Read the model definition and answer for the solid it produces. Units are mm, in the model's axes. Face numbers are marked on the shaded views. A direction names the side the tool comes from. Give positions to 0.01 mm unless a question says otherwise; leave off trailing zeros. Order: outer loops, then holes, each group sorted by start corner. A loop starts at its lowest first (then second) coordinate and runs counter-clockwise, first axis right, second up.
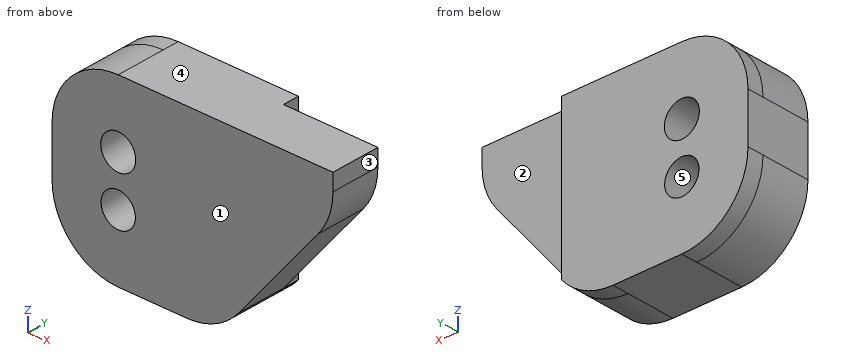
```python
from build123d import *

# Parameters (mm, degrees)
BOSS_EXTRUDE1_DEPTH = 19.05
FILLET1_R           = 25.4
BOSS_EXTRUDE2_DEPTH = 6.35
SKETCH4_R           = 6.721788933
SKETCH4_R_2         = 6.590945077
CUT_EXTRUDE3_DEPTH  = 26.4


with BuildPart() as part:
    # Sketch1 → Boss-Extrude1 (new body)
    with BuildSketch(Plane(origin=(0, 0, 0), x_dir=(1, 0, 0), z_dir=(0, 1, 0))):
        Polygon((10.04026689, 34.907603773), (53.917892581, -19.499033471), (53.917892581, -34.907603773), (-53.917892581, -34.907603773), (-53.917892581, 34.907603773), align=None)
    extrude(amount=BOSS_EXTRUDE1_DEPTH)

    # Fillet1
    fillet1_edges = [part.edges().sort_by_distance(p)[0] for p in [
        (-53.917892581, 9.525, -34.907603773),
        (10.04026689, 9.525, -34.907603773),
        (53.917892581, 9.525, 19.499033471),
        (-53.917892581, 9.525, 34.907603773),
    ]]
    fillet(fillet1_edges, radius=FILLET1_R)

    # Sketch3 → Boss-Extrude2 (add)
    with BuildSketch(Plane(origin=(0, 19.05, 0), x_dir=(1, 0, 0), z_dir=(0, 1, 0))):
        with BuildLine():
            Line((17.665332694, 25.452803459), (17.665332694, -34.907603773))
            Line((17.665332694, -34.907603773), (-28.517892581, -34.907603773))
            ThreePointArc((-28.517892581, -34.907603773), (-46.478404823, -27.468116015), (-53.917892581, -9.507603773))
            Line((-53.917892581, -9.507603773), (-53.917892581, 9.507603773))
            ThreePointArc((-53.917892581, 9.507603773), (-46.478404823, 27.468116015), (-28.517892581, 34.907603773))
            Line((-28.517892581, 34.907603773), (-2.106126711, 34.907603773))
            ThreePointArc((-2.106126711, 34.907603773), (8.851791157, 32.422315991), (17.665332694, 25.452803459))
        make_face()
    extrude(amount=BOSS_EXTRUDE2_DEPTH)

    # Sketch4 → Cut-Extrude3 (cut, through all)
    with BuildSketch(Plane(origin=(0, 25.4, 0), x_dir=(1, 0, 0), z_dir=(0, 1, 0))):
        with Locations(Location((-28.517892581, -9.507603773, 0), (0, 0, 270))):  # turned: the seam where the file's is
            Circle(SKETCH4_R)
        with Locations(Location((-28.517892581, 9.507603773, 0), (0, 0, 270))):  # turned: the seam where the file's is
            Circle(SKETCH4_R_2)
    extrude(amount=-CUT_EXTRUDE3_DEPTH, mode=Mode.SUBTRACT)


solid = part.part
```
1) The part is cut by section B-B on z = 19.5. Determine the outline of the cut face in (x, y), and give its area (3 significant figures).
Final values:
outline: (-51.87, 0) - (52.28, 0) - (52.28, 19.05) - (17.67, 19.05) - (17.67, 25.4) - (-51.87, 25.4) - close
area: 2,430 mm2
2) Given pin 1 (11 mm diameter, centred on x = 39.5, z = 5.5, fed in from +Y); pin 2 (1.9 mm diameter, centred on y = 21.5, z = 8, fed in from +X); pin 3 (12 mm diameter, centred on x = -28.52, z = 9.51, fed in from +Y); pin 4 (2 mm diameter, centred on y = 7, z = 22, fed in from +X), each flat-ended and moving along its own axis, determine where each tip first touches the part or whether it passes through.
Final values:
pin 1: stops at y = 19.05
pin 2: stops at x = 17.67
pin 3: passes through
pin 4: stops at x = 53.32
3) The part is cut by section C-C on x = 13. Determine the outline of the cut face in (y, z), and give its area (3 significant figures).
Final values:
outline: (0, -29.93) - (25.4, -29.93) - (25.4, 34.91) - (0, 34.91) - close
area: 1,650 mm2
4) The part is cut by section A-A on y = 2. Determine the outline of the cut face in (x, z), and give its area (3 significant figures).
Final values:
outline: (-53.92, -9.51) arc R25.4 ccw to (-28.52, -34.91) - (-2.11, -34.91) arc R25.4 ccw to (17.67, -25.45) - (48.29, 12.52) arc R25.4 ccw to (53.92, 28.47) - (53.92, 34.91) - (-28.52, 34.91) arc R25.4 ccw to (-53.92, 9.51) - close; hole circle Ø13.44 at (-28.52, 9.51); hole circle Ø13.18 at (-28.52, -9.51)
area: 5,750 mm2
5) The part is cut by section D-D on y = 23.75. Determine the outline of the cut face in (x, z).
Final values:
outline: (-53.92, -9.51) arc R25.4 ccw to (-28.52, -34.91) - (-2.11, -34.91) arc R25.4 ccw to (17.67, -25.45) - (17.67, 34.91) - (-28.52, 34.91) arc R25.4 ccw to (-53.92, 9.51) - close; hole circle Ø13.44 at (-28.52, 9.51); hole circle Ø13.18 at (-28.52, -9.51)
6) For a pull along Z with two mould halves and no side action, classify the marked faces 3, 4 and 5 as released by +Z, released by -Z, zero draft, split by the parting line, or undercut.
Final values:
face 3: zero draft
face 4: released by +Z
face 5: undercut
7) Consider L1, parallel to Y at x = 25.5, z = 32.5; L2, parallel to X at y = 6.25, z = 13.5; L3, parallel to X at y = 9, z = 15. Determine where each line is inside the solid, lowest interval first.
Final values:
L1: y = 0 to 19.05
L2: x = -53.6 to -33.93, -23.11 to 49.04
L3: x = -53.32 to -32.39, -24.64 to 50.06
8) A tool of negligible diameter and unlimited length cuts with its end or side. For the marked faces 1 and 2, from which of +Z, -Z, +X, -X, +Y, -Y can it reach the whole face along a straight path? Write none if from no direction.
Final values:
face 1: +Z, -Z, +X, -X, -Y
face 2: +Z, -Z, +X, +Y
